```python
from build123d import *

# Parameters (mm, degrees)
F0_W     = 2.5
F0_H     = 23
F0_W_2   = 23
F0_H_2   = 2.5
F1_DEPTH = 3


with BuildPart() as f1:
    # F0 (on Top) → F1 (new body)
    with BuildSketch(Plane.XY):
        Polygon((-112.64636, -2.5), (-112.64636, -77.5), (-102.64636, -77.5), (-79.64636, -77.5), (104.35364, -77.5), (127.35364, -77.5), (137.35364, -77.5), (137.35364, -2.5), (127.35364, -2.5), (104.35364, -2.5), (-79.64636, -2.5), (-102.64636, -2.5), align=None)
        with Locations((-108.39636, -40)):
            Rectangle(F0_W, F0_H, mode=Mode.SUBTRACT)
        with Locations((-91.14636, -78.75)):
            Rectangle(F0_W_2, F0_H_2)
        with Locations((-91.14636, -1.25)):
            Rectangle(F0_W_2, F0_H_2)
        with Locations((115.85364, -78.75)):
            Rectangle(F0_W_2, F0_H_2)
        with Locations((115.85364, -1.25)):
            Rectangle(F0_W_2, F0_H_2)
    extrude(amount=F1_DEPTH)


solid = f1.part
```
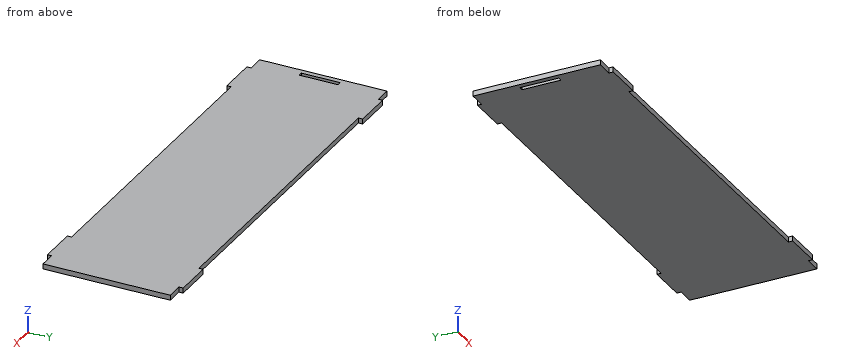
Design review of the part built by this model. Coordinates are the model's own, in mm. Coordinates: 2 decimals unless noted, no trailing zeros. Loops run counter-clockwise (first coordinate to the right, second up) from the corner with the lowest first, then second, coordinate; pieces in that order, holes last. Notation, with made-up numbers: (-29.75, 22.25) -> (-20.75, 22.25) arc R33 cw to (-20.75, 58.25) -> close; hole circle Ø8 at (77, 14.25). An arc over 180 degrees is marked (long way). Answer as a JSON object with one key per item and string values.
Q1. Clearance check with flat-ended pins moving along their axes: pin 1 Ø1.5 at (x, z) = (-107.5, 1) entering from -Y; pin 2 Ø0.8 at (y, z) = (-78, 2) entering from +X; pin 3 Ø0.8 at (y, z) = (-78.5, 1) entering from -X. State where each tip first meets the part, or that it passes through.
Answer block:
{"pin 1": "stops at y = -77.5", "pin 2": "stops at x = 127.35", "pin 3": "stops at x = -102.65"}
Q2. Take a section at A-A on z = 1.3. Give the boundary of the cut face in (x, y).
Answer block:
{"outline": "(-112.65, -77.5) -> (-102.65, -77.5) -> (-102.65, -80) -> (-79.65, -80) -> (-79.65, -77.5) -> (104.35, -77.5) -> (104.35, -80) -> (127.35, -80) -> (127.35, -77.5) -> (137.35, -77.5) -> (137.35, -2.5) -> (127.35, -2.5) -> (127.35, 0) -> (104.35, 0) -> (104.35, -2.5) -> (-79.65, -2.5) -> (-79.65, 0) -> (-102.65, 0) -> (-102.65, -2.5) -> (-112.65, -2.5) -> close; hole (-109.65, -51.5) -> (-107.15, -51.5) -> (-107.15, -28.5) -> (-109.65, -28.5) -> close"}
Q3. To check wall thickness, follow L1, parallel to X at y = -46, z = 2.65; L2, parallel to Y at x = 91, z = 0.75. State the ranges of each line that lie inside material, in increasing order.
Answer block:
{"L1": "x = -112.65 to -109.65, -107.15 to 137.35", "L2": "y = -77.5 to -2.5"}
Q4. Take a section at B-B on x = 44. Give the boundary of the cut face in (y, z), plus the area to 3 significant figures.
Answer block:
{"outline": "(-77.5, 0) -> (-2.5, 0) -> (-2.5, 3) -> (-77.5, 3) -> close", "area": "225 mm^2"}
